```python
from build123d import *

# Parameters (mm, degrees)
SKETCH_1_W               = 30
SKETCH_1_H               = 15
EXTRUDE_1_DEPTH          = 18
CUT_EXTRUDE_1_REACH      = 28.843
SKETCH_2_W               = 20
SKETCH_2_H               = 10
CUT_EXTRUDE_2_REACH      = 29.668
SKETCH_3_W               = 20
SKETCH_3_H               = 12
CUT_EXTRUDE_5_DEPTH      = 22.1
CUT_EXTRUDE_5_DEPTH_BACK = 2.1
SKETCH_4_W               = 5
SKETCH_4_H               = 6
SKETCH_5_R               = 2.5
EXTRUDE_2_DEPTH          = 1.6
EXTRUDE_START            = 1.6
SKETCH_6_R               = 2.5
EXTRUDE_3_DEPTH          = 1.6
CHAMFER_1_SIZE           = 0.4
CUT_EXTRUDE_6_DEPTH      = 35.020684023
CUT_EXTRUDE_6_DEPTH_BACK = 35.020684023
CUT_EXTRUDE_7_DEPTH      = 35.020684023
CUT_EXTRUDE_7_DEPTH_BACK = 35.020684023
EXTRUDE_4_DEPTH          = 20
SKETCH_10_R              = 2.6
CUT_EXTRUDE_8_DEPTH      = 35.965796737
CUT_EXTRUDE_9_DEPTH      = 35.965796737
CUT_EXTRUDE_9_DEPTH_BACK = 35.965796737
SKETCH_12_W              = 1.696031958
SKETCH_12_H              = 15
CHAMFER_2_SIZE           = 2
SKETCH_17_W              = 3.1
SKETCH_17_H              = 15
EXTRUDE_8_DEPTH          = 0.27


with BuildPart() as part:
    # 草圖1 → 填料-伸長1 (new body)
    with BuildSketch(Plane.XY):
        with Locations((2.249045701, -2.44972067)):
            Rectangle(SKETCH_1_W, SKETCH_1_H)
    extrude(amount=EXTRUDE_1_DEPTH)

    # 草圖2 → 除料-伸長1 (cut, up to next)
    with BuildSketch(Plane.XY.offset(18), mode=Mode.PRIVATE) as cut_extrude_1_sk1:
        with Locations((2.249045701, -1.94972067)):
            Rectangle(SKETCH_2_W, SKETCH_2_H)
    cut_extrude_1_tool1 = extrude(cut_extrude_1_sk1.sketch, amount=-CUT_EXTRUDE_1_REACH, mode=Mode.PRIVATE) & part.part
    add(cut_extrude_1_tool1.solids().sort_by_distance((2.249046, -1.949721, 18))[0], mode=Mode.SUBTRACT)

    # 草圖3 → 除料-伸長2 (cut, up to next)
    with BuildSketch(Plane(origin=(0, -6.94972067, 0), x_dir=(1, 0, 0), z_dir=(0, 1, 0)), mode=Mode.PRIVATE) as cut_extrude_2_sk1:
        with Locations((2.249045701, -12)):
            Rectangle(SKETCH_3_W, SKETCH_3_H)
    cut_extrude_2_tool1 = extrude(cut_extrude_2_sk1.sketch, amount=-CUT_EXTRUDE_2_REACH, mode=Mode.PRIVATE) & part.part
    add(cut_extrude_2_tool1.solids().sort_by_distance((2.249046, -6.949721, 12))[0], mode=Mode.SUBTRACT)

    # 草圖4 → 除料-伸長5 (cut, two sides: drawn at the far end of the back side and taken through both)
    with BuildSketch(Plane(origin=(-7.750954299, 0, 0), x_dir=(0, 0, -1), z_dir=(1, 0, 0)).offset(-CUT_EXTRUDE_5_DEPTH_BACK)):
        with Locations((-15.5, 0.05027933)):
            Rectangle(SKETCH_4_W, SKETCH_4_H)
        with BuildLine():
            Line((-13, 3.05027933), (-13, -2.94972067))
            Line((-13, -2.94972067), (-18, -2.94972067))
            Line((-18, -2.94972067), (-18, -9.94972067))
            Line((-18, -9.94972067), (-6, -9.94972067))
            Line((-6, -9.94972067), (-6, -6.94972067))
            Line((-6, -6.94972067), (-3.562706956, -6.94972067))
            ThreePointArc((-3.562706956, -6.94972067), (-2.955231369, -4.990584005), (-2.75, -2.94972067))
            ThreePointArc((-2.75, -2.94972067), (-3.246950555, 0.203139384), (-4.689614931, 3.05027933))
            Line((-4.689614931, 3.05027933), (-13, 3.05027933))
        make_face()
        with BuildLine():
            ThreePointArc((-18, 5.998044414), (-15.583399687, 6.969379392), (-13, 7.30027933))
            Line((-13, 7.30027933), (-13, 7.89449882))
            Line((-13, 7.89449882), (-18, 7.89449882))
            Line((-18, 7.89449882), (-18, 5.998044414))
        make_face()
        with BuildLine():
            Line((-13, 7.30027933), (-13, 3.05027933))
            Line((-13, 3.05027933), (-4.689614931, 3.05027933))
            ThreePointArc((-4.689614931, 3.05027933), (-8.332961324, 6.176135454), (-13, 7.30027933))
        make_face()
        with BuildLine():
            Line((-18, 3.05027933), (-13, 3.05027933))
            Line((-13, 3.05027933), (-13, 7.30027933))
            ThreePointArc((-13, 7.30027933), (-15.583399687, 6.969379392), (-18, 5.998044414))
            Line((-18, 5.998044414), (-18, 3.05027933))
        make_face()
        with BuildLine():
            Line((-18, -9.94972067), (-18, -2.94972067))
            Line((-18, -2.94972067), (-18, 3.05027933))
            Line((-18, 3.05027933), (-18, 5.998044414))
            ThreePointArc((-18, 5.998044414), (-19.843504041, -10.580510436), (-3.562706956, -6.94972067))
            Line((-3.562706956, -6.94972067), (-6, -6.94972067))
            Line((-6, -6.94972067), (-6, -9.94972067))
            Line((-6, -9.94972067), (-18, -9.94972067))
        make_face()
    extrude(amount=CUT_EXTRUDE_5_DEPTH + CUT_EXTRUDE_5_DEPTH_BACK, mode=Mode.SUBTRACT)

    # 草圖5 → 填料-伸長2 (add)
    with BuildSketch(Plane.ZY.offset(-14.349045701)):
        with Locations(Location((13, -2.94972067, 0), (0, 0, 90))):
            Circle(SKETCH_5_R)
    extrude(amount=EXTRUDE_2_DEPTH)

    # 草圖6 → 填料-伸長3 (add)
    with BuildSketch(Plane(origin=(-9.850954299, 0, 0), x_dir=(0, 0, -1), z_dir=(1, 0, 0)).offset(EXTRUDE_START)):
        with Locations(Location((-13, -2.94972067, 0), (0, 0, 90))):
            Circle(SKETCH_6_R)
    extrude(amount=-EXTRUDE_3_DEPTH)

    # 導角1
    chamfer_1_edges = [part.edges().sort_by_distance(p)[0] for p in [
        (12.749045701, -5.44972067, 13),
        (-8.250954299, -5.44972067, 13),
    ]]
    chamfer(chamfer_1_edges, length=CHAMFER_1_SIZE)

    # 草圖7 → 除料-伸長6 (cut, two sides: drawn at the far end of the back side and taken through both)
    with BuildSketch(Plane(origin=(-9.850954299, 0, 0), x_dir=(0, 0, -1), z_dir=(1, 0, 0)).offset(-CUT_EXTRUDE_6_DEPTH_BACK)):
        Polygon((-18, -9.94972067), (-13.071067812, -9.94972067), (-18, -5.020788482), align=None)
    extrude(amount=CUT_EXTRUDE_6_DEPTH + CUT_EXTRUDE_6_DEPTH_BACK, mode=Mode.SUBTRACT)

    # 草圖8 → 除料-伸長7 (cut, two sides: drawn at the far end of the back side and taken through both)
    with BuildSketch(Plane(origin=(-9.850954299, 0, 0), x_dir=(0, 0, -1), z_dir=(1, 0, 0)).offset(-CUT_EXTRUDE_7_DEPTH_BACK)):
        with BuildLine():
            Line((-18, -2.94972067), (-18, -5.020788482))
            Line((-18, -5.020788482), (-16.535533871, -6.485254612))
            ThreePointArc((-16.535533871, -6.485254612), (-17.619397653, -4.863137855), (-18, -2.94972067))
        make_face()
    extrude(amount=CUT_EXTRUDE_7_DEPTH + CUT_EXTRUDE_7_DEPTH_BACK, mode=Mode.SUBTRACT)

    # 草圖9 → 填料-伸長4 (add)
    with BuildSketch(Plane(origin=(0, 0, 0), x_dir=(-1, 0, 0), z_dir=(0, 0, -1))):
        Polygon((9.650954299, 5.05027933), (7.750954299, 5.05027933), (7.750954299, 3.05027933), (7.750954299, -6.94972067), (7.750954299, -9.94972067), (9.650954299, -9.94972067), align=None)
        Polygon((-12.249045701, 3.05027933), (-12.249045701, 5.05027933), (-14.149045701, 5.05027933), (-14.149045701, -9.94972067), (-12.249045701, -9.94972067), (-12.249045701, -6.94972067), align=None)
    extrude(amount=EXTRUDE_4_DEPTH)

    # 草圖10 → 除料-伸長8 (cut, through all)
    with BuildSketch(Plane(origin=(14.149045701, 0, 0), x_dir=(0, 0, -1), z_dir=(1, 0, 0))):
        with Locations((5.2, -2.94972067)):
            Circle(SKETCH_10_R)
    extrude(amount=-CUT_EXTRUDE_8_DEPTH, mode=Mode.SUBTRACT)

    # 草圖12 → 除料-伸長9 (cut, two sides: drawn at the far end of the back side and taken through both)
    with BuildSketch(Plane(origin=(14.149045701, 0, 0), x_dir=(0, 0, -1), z_dir=(1, 0, 0)).offset(-CUT_EXTRUDE_9_DEPTH_BACK)):
        with BuildLine():
            Line((18.303968042, 5.05027933), (5.2, 5.05027933))
            ThreePointArc((5.2, 5.05027933), (10.856854249, 2.707133579), (13.2, -2.94972067))
            ThreePointArc((13.2, -2.94972067), (12.091439137, -7.012732683), (9.072983346, -9.94972067))
            Line((9.072983346, -9.94972067), (18.303968042, -9.94972067))
            Line((18.303968042, -9.94972067), (18.303968042, 5.05027933))
        make_face()
        with Locations((19.151984021, -2.44972067)):
            Rectangle(SKETCH_12_W, SKETCH_12_H)
    extrude(amount=CUT_EXTRUDE_9_DEPTH + CUT_EXTRUDE_9_DEPTH_BACK, mode=Mode.SUBTRACT)

    # 導角2
    chamfer_2_edges = [part.edges().sort_by_distance(p)[0] for p in [
        (15.799045701, 5.05027933, 18),
        (-11.300954299, 5.05027933, 18),
    ]]
    chamfer(chamfer_2_edges, length=CHAMFER_2_SIZE)

    # 草圖17 → 填料-伸長8 (add)
    with BuildSketch(Plane(origin=(0, 0, 0), x_dir=(-1, 0, 0), z_dir=(0, 0, -1))):
        with Locations((-15.699045701, -2.44972067)):
            Rectangle(SKETCH_17_W, SKETCH_17_H)
        with Locations((11.200954299, -2.44972067)):
            Rectangle(SKETCH_17_W, SKETCH_17_H)
    extrude(amount=EXTRUDE_8_DEPTH)


solid = part.part
```
Work out the finished part from the listing and answer in its coordinate system (mm). A direction names the side the tool comes from. Give positions to 0.01 mm unless a question says otherwise; leave off trailing zeros. Order: outer loops, then holes, each group sorted by start corner. A loop starts at its lowest first (then second) coordinate and runs counter-clockwise, first axis right, second up. Notation, with made-up numbers: (70.25, 29.25) - (74.25, 29.25) arc R25 ccw to (74.25, 42.25) - close; hole circle Ø6 at (-10, 25). An arc over 180 degrees is marked (long way). One line per item, written item: value. Start each with the question number.
1. Each of these flat-tipped pins is pushed along its axis until it touches: pin 1 Ø6.5 at (y, z) = (-2, -5) entering from -X; pin 2 Ø3 at (x, y) = (10.5, -7.5) entering from +Z; pin 3 Ø2.5 at (x, y) = (16.5, 0) entering from -Z. Where does it stop, or does it pass through?
2. Which of the six approach directions +Z, -Z, +X, -X, +Y, -Y give full straight-line access (tool end or side, diameter ignored) to faces 5 (the face through (-9.24, -3.49, 10.56)), 6 (the face through (16, -2, -0.27)), 7 (the face through (12.749, -3, 13))?
3. Section B-B, the plane x = 9 is taken. Write down the section's boundary in (y, z).
4. For a pull along X with two mould halves and no side action, classify faces 1 (the face through (15.78, -4.89, 17.61)), 2 (the face through (-9.851, -2, 10)), 3 (the face through (2, 4, 0)), 4 (the face through (-9.651, -3, -8)) as released by +X, released by -X, zero draft, split by the parting line, or undercut.
5. Section A-A, the plane z = 2 is taken. Write down the section's boundary in (x, y).
6. Section D-D, the plane z = -3 is taken. Write down the section's boundary in (x, y).
7. Section C-C, the plane y = 1 is taken. Write down the section's boundary in (x, z), then the cut area to 3 significant figures.
8. Consider line 1 (X direction, y = -8.25, z = -4); line 2 (Y direction, x = 12.75, z = -5.2); line 3 (X direction, y = -3, z = 16). Determine where each line is inside the solid, lowest interval first.
Filled sheet:
1. pin 1: x = -9.65
1. pin 2: z = 4.73
1. pin 3: z = -0.27
2. face 5: none
2. face 6: -Z, +X, +Y, -Y
2. face 7: +Z, +Y, -Y
3. outline: (-9.95, 0) - (-6.95, 0) - (-6.95, 3.56) arc R10.25 cw to (-9.95, 5.51) - close; (3.05, 0) - (5.05, 0) - (5.05, 6.59) arc R10.25 cw to (3.05, 4.69) - close
4. face 1: zero draft
4. face 2: undercut
4. face 3: undercut
4. face 4: released by -X
5. outline: (-12.75, -9.95) - (17.25, -9.95) - (17.25, 5.05) - (-12.75, 5.05) - close; hole (-7.75, -6.95) - (12.25, -6.95) - (12.25, 3.05) - (-7.75, 3.05) - close
6. outline: (-9.65, -9.95) - (-7.75, -9.95) - (-7.75, -4.34) - (-9.65, -4.34) - close; (-9.65, -1.56) - (-7.75, -1.56) - (-7.75, 5.05) - (-9.65, 5.05) - close; (12.25, -9.95) - (14.15, -9.95) - (14.15, -4.34) - (12.25, -4.34) - close; (12.25, -1.56) - (14.15, -1.56) - (14.15, 5.05) - (12.25, 5.05) - close
7. outline: (-12.75, -0.27) - (-9.65, -0.27) - (-9.65, -12.16) - (-7.75, -12.16) - (-7.75, 3.54) - (-9.85, 3.54) - (-9.85, 18) - (-12.75, 18) - close; (12.25, -12.16) - (14.15, -12.16) - (14.15, -0.27) - (17.25, -0.27) - (17.25, 18) - (14.35, 18) - (14.35, 3.54) - (12.25, 3.54) - close
7. area: 167 mm²
8. line 1: -9.65 to -7.75, 12.25 to 14.15
8. line 2: -9.95 to -5.55, -0.35 to 5.05
8. line 3: -12.75 to -9.85, 14.35 to 17.25
